Here's how the part is built. I have some questions about the finished solid (model axes, mm). A direction names the side the tool comes from. Give positions to 0.01 mm unless a question says otherwise; leave off trailing zeros. Order: outer loops, then holes, each group sorted by start corner. A loop starts at its lowest first (then second) coordinate and runs counter-clockwise, first axis right, second up. Notation, with made-up numbers: (86, -28) - (144, -28) arc R18 cw to (144, -17) - close; hole circle Ø5 at (80, 71.5). An arc over 180 degrees is marked (long way). One line per question, with ' | ' between items.
from build123d import *

# Parameters (mm, degrees)
SKETCH1_W           = 100
SKETCH1_H           = 60
SKETCH1_R           = 20
BOSS_EXTRUDE1_DEPTH = 60
BOSS_EXTRUDE2_DEPTH = 30
BOSS_EXTRUDE3_DEPTH = 50
CUT_EXTRUDE1_DEPTH  = 61


with BuildPart() as part:
    # Sketch1 → Boss-Extrude1 (new body)
    with BuildSketch(Plane(origin=(0, 0, 0), x_dir=(1, 0, 0), z_dir=(0, 1, 0))):
        Rectangle(SKETCH1_W, SKETCH1_H)
        Circle(SKETCH1_R, mode=Mode.SUBTRACT)
    extrude(amount=BOSS_EXTRUDE1_DEPTH)

    # Sketch3 → Boss-Extrude2 (add, symmetric)
    with BuildSketch(Plane.XY):
        Polygon((50, 0), (50, 50), (110, 0), align=None)
        Polygon((-110, 0), (-50, 0), (-50, 50), align=None)
    extrude(amount=BOSS_EXTRUDE2_DEPTH, both=True)

    # Sketch4 → Boss-Extrude3 (add, symmetric)
    with BuildSketch(Plane(origin=(0, 0, 0), x_dir=(0, 0, -1), z_dir=(1, 0, 0))):
        Polygon((-30, 0), (-30, 50), (-70, 0), align=None)
        Polygon((30, 0), (30, 50), (70, 0), align=None)
    extrude(amount=BOSS_EXTRUDE3_DEPTH, both=True)

    # Sketch5 → Cut-Extrude1 (cut, through all)
    with BuildSketch(Plane(origin=(0, 0, 0), x_dir=(1, 0, 0), z_dir=(0, 1, 0))):
        Polygon((-40, -70), (0, -40), (40, -70), align=None)
        Polygon((0, 40), (40, 70), (-40, 70), align=None)
        Polygon((110, -20), (70, 0), (110, 20), align=None)
        Polygon((-110, 20), (-110, -20), (-70, 0), align=None)
    extrude(amount=CUT_EXTRUDE1_DEPTH, mode=Mode.SUBTRACT)


solid = part.part
1) I'm going to push flat-ended pins straight in: P1, Ø20, axis at y = 14.5, z = 43, coming from the +X side; P2, Ø4, axis at x = -43.5, y = 30, coming from the +Z side; P3, Ø3, axis at x = -22, y = 40.5, coming from the +Z side; P4, Ø24, axis at x = 0, z = 0, coming from the +Y side. Where does each tip first touch, or does it pass through?
Model answer:
P1: stops at x = 50 | P2: stops at z = 47.6 | P3: stops at z = 38.8 | P4: passes through
2) Please list where these lines run through material, in increasing order: L1, parallel to X at y = 16, z = 0; L2, parallel to Z at x = 0, y = 13; L3, parallel to Z at x = 0, y = 44.
Model answer:
L1: x = -70 to -20, 20 to 70 | L2: z = -40 to -20, 20 to 40 | L3: z = -34.8 to -20, 20 to 34.8
3) I want a section at A-A (x = 77). List the corners of the cut face in (y, z) for me, plus the area to 3 significant figures.
Model answer:
outline: (0, -30) - (27.5, -30) - (27.5, -3.5) - (0, -3.5) - close; (0, 3.5) - (27.5, 3.5) - (27.5, 30) - (0, 30) - close | area: 1,460 mm2
4) Thinking about a two-plate mould opening in Z: for faces 1 (the face through (11.811, 30.906, -45.276)), 2 (the face through (-11.811, 30.906, 45.276)), 3 (the face through (81.4, 9, 5.7)), 4 (the face through (85.28, 12.73, -7.64)), which applies, +Z half, -Z half, draft (parallel to the pull), parting line (faces both ways), or undercut?
Model answer:
face 1: -Z half | face 2: +Z half | face 3: undercut | face 4: undercut
5) I want a section at D-D (z = -56). List the corners of the cut face in (x, y) for me, plus the area to 3 significant figures.
Model answer:
outline: (-50, 0) - (-21.33, 0) - (-21.33, 17.5) - (-50, 17.5) - close; (21.33, 0) - (50, 0) - (50, 17.5) - (21.33, 17.5) - close | area: 1,000 mm2
6) On a 3-axis mill with a long thin cutter (end or side, diameter ignored), from which of +Z, -Z, +X, -X, +Y, -Y can I reach the whole of each face in a straight line? I mean faces 5 (the face through (-81.4, 9, 5.7)), 6 (the face through (15.28, 14.32, -51.46)), 7 (the face through (50, 14, -41)), 8 (the face through (-1, 55, -30)). Say none if no direction works.
Model answer:
face 5: -X, +Y, -Y | face 6: -Z, +Y, -Y | face 7: -Z, +X, +Y, -Y | face 8: -Z, +X, -X, +Y
7) I want a section at C-C (z = -27). List the corners of the cut face in (x, y) for me.
Model answer:
outline: (-110, 0) - (110, 0) - (50, 50) - (50, 60) - (-50, 60) - (-50, 50) - close
8) I want a section at B-B (y = 10.5). List the corners of the cut face in (x, z) for me, plus the area to 3 significant figures.
Model answer:
outline: (-97.4, -30) - (-50, -30) - (-50, -61.6) - (-28.8, -61.6) - (0, -40) - (28.8, -61.6) - (50, -61.6) - (50, -30) - (97.4, -30) - (97.4, -13.7) - (70, 0) - (97.4, 13.7) - (97.4, 30) - (50, 30) - (50, 61.6) - (28.8, 61.6) - (0, 40) - (-28.8, 61.6) - (-50, 61.6) - (-50, 30) - (-97.4, 30) - (-97.4, 13.7) - (-70, 0) - (-97.4, -13.7) - close; hole circle Ø40 at (0, 0) | area: 14,800 mm2
